```python
from build123d import *

# Parameters (mm, degrees)
SKETCH_1_W          = 6.6
SKETCH_1_H          = 1.5
SKETCH_1_W_2        = 1.6
SKETCH_2_R          = 2
CUT_EXTRUDE_1_DEPTH = 5


with BuildPart() as part:
    # 草图1 → 旋转2 (revolve)
    with BuildSketch(Plane.XY):
        with Locations((-25.652830189, 0.75)):
            Rectangle(SKETCH_1_W, SKETCH_1_H)
        Polygon((-22.352830189, 1.5), (-22.352830189, 0), (-19.352830189, 0), (-19.352830189, 4.55), (-22.352830189, 4.55), align=None)
        Polygon((-19.352830189, 4.55), (-19.352830189, 0), (2.247169811, 0), (2.247169811, 4.55), (2.247169811, 17.65), (-19.352830189, 17.65), align=None)
        Polygon((2.247169811, 4.55), (2.247169811, 0), (6.047169811, 0), (6.047169811, 1.5), (6.047169811, 4.55), align=None)
        with Locations((6.847169811, 0.75)):
            Rectangle(SKETCH_1_W_2, SKETCH_1_H)
    revolve(axis=Axis((-28.952830189, 0, 0), (1, 0, 0)))

    # 草图2 → 切除-拉伸1 (cut)
    with BuildSketch(Plane.ZY.offset(19.352830189)):
        with Locations((0, 12.5)):
            Circle(SKETCH_2_R)
        with Locations((0, -12.5)):
            Circle(SKETCH_2_R)
        with Locations((-12.5, 0)):
            Circle(SKETCH_2_R)
        with Locations((12.5, 0)):
            Circle(SKETCH_2_R)
    extrude(amount=-CUT_EXTRUDE_1_DEPTH, mode=Mode.SUBTRACT)


solid = part.part
```
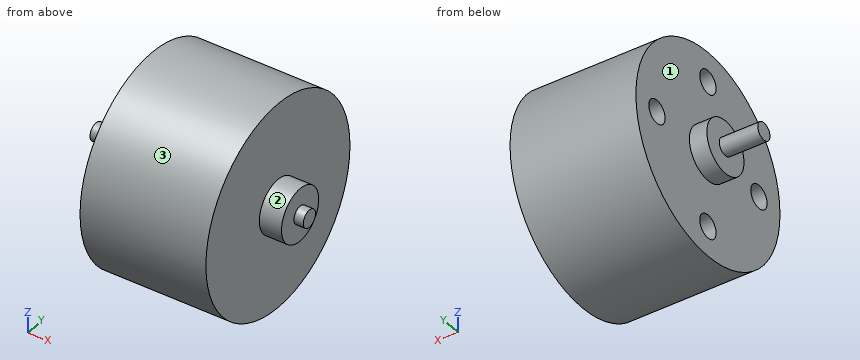
The model under review builds one solid part; all positions refer to its coordinate system, in mm. Face numbers are marked on the shaded views. A direction names the side the tool comes from. Give positions to 0.01 mm unless a question says otherwise; leave off trailing zeros. Order: outer loops, then holes, each group sorted by start corner. A loop starts at its lowest first (then second) coordinate and runs counter-clockwise, first axis right, second up. Notation, with made-up numbers: (46.5, 71.25) - (66.5, 71.25) arc R26 cw to (66.5, 103.25) - close; hole circle Ø10 at (57, -15). An arc over 180 degrees is marked (long way). Use CSV: the item, a comma, the result in double quotes. Start each with the question number.
Q1. We need section D-D, the plane y = -12.5. Write out the cut boundary in (x, z), and give its area (3 significant figures).
Q2. We need section C-C, the plane x = -23.5. Write out the cut boundary in (y, z).
Q3. We need section A-A, the plane y = 0. Write out the cut boundary in (x, z), and give its area (3 significant figures).
Q4. To check wall thickness, follow line 1 along Z through (x, y) = (-17, -0.5); line 2 along Y through (x, z) = (-17.5, 12); line 3 along X through (y, z) = (-9, -4.5). State the ranges of each line that lie inside material, in increasing order. Write a range as [from, to].
Q5. Tool access review of the marked faces 1, 2 and 3: name each direction out of +Z, -Z, +X, -X, +Y, -Y from which nothing blocks a thin tool from reaching the whole face with its end or side.
Q6. Clearance check with flat-ended pins moving along their axes: pin 1 Ø2 at (y, z) = (-13, 0) entering from -X; pin 2 Ø8 at (x, y) = (-15, 13.5) entering from -Z; pin 3 Ø3 at (y, z) = (-12.5, 0) entering from +X; pin 4 Ø12 at (y, z) = (1, 2) entering from +X. State where each tip first meets the part, or that it passes through.
Outcome:
1,outline,"(-19.35, -12.46) - (2.25, -12.46) - (2.25, 12.46) - (-19.35, 12.46) - (-19.35, 2) - (-14.35, 2) - (-14.35, -2) - (-19.35, -2) - close"
1,area,"518 mm^2"
2,outline,"circle Ø3 at (0, 0)"
3,outline,"(-28.95, -1.5) - (-22.35, -1.5) - (-22.35, -4.55) - (-19.35, -4.55) - (-19.35, -10.5) - (-14.35, -10.5) - (-14.35, -14.5) - (-19.35, -14.5) - (-19.35, -17.65) - (2.25, -17.65) - (2.25, -4.55) - (6.05, -4.55) - (6.05, -1.5) - (7.65, -1.5) - (7.65, 1.5) - (6.05, 1.5) - (6.05, 4.55) - (2.25, 4.55) - (2.25, 17.65) - (-19.35, 17.65) - (-19.35, 14.5) - (-14.35, 14.5) - (-14.35, 10.5) - (-19.35, 10.5) - (-19.35, 4.55) - (-22.35, 4.55) - (-22.35, 1.5) - (-28.95, 1.5) - close"
3,area,"809 mm^2"
4,line 1,"z = [-17.64, -14.44], [-10.56, 10.56], [14.44, 17.64]"
4,line 2,"y = [-12.94, -1.94], [1.94, 12.94]"
4,line 3,"x = [-19.35, 2.25]"
5,face 1,"-X"
5,face 2,"+X"
5,face 3,"+X, -X"
6,pin 1,"stops at x = -14.35"
6,pin 2,"stops at z = -14.88"
6,pin 3,"stops at x = 2.25"
6,pin 4,"stops at x = 7.65"
